Geometry: see drawing. Coordinates: mm, zero at the bounding-box minimum. A direction names the side the tool comes from. Round coordinates to 2 decimals unless told otherwise and drop trailing zeros. Loops run counter-clockwise (first coordinate to the right, second up) from the corner with the lowest first, then second, coordinate; pieces in that order, holes last. Notation, with made-up numbers: (72, 47.5) -> (87, 47.5) arc R8 ccw to (87, 61.5) -> close; hole circle Ø1 at (32.25, 64). An arc over 180 degrees is marked (long way). Answer in a Markdown table with one row per item.
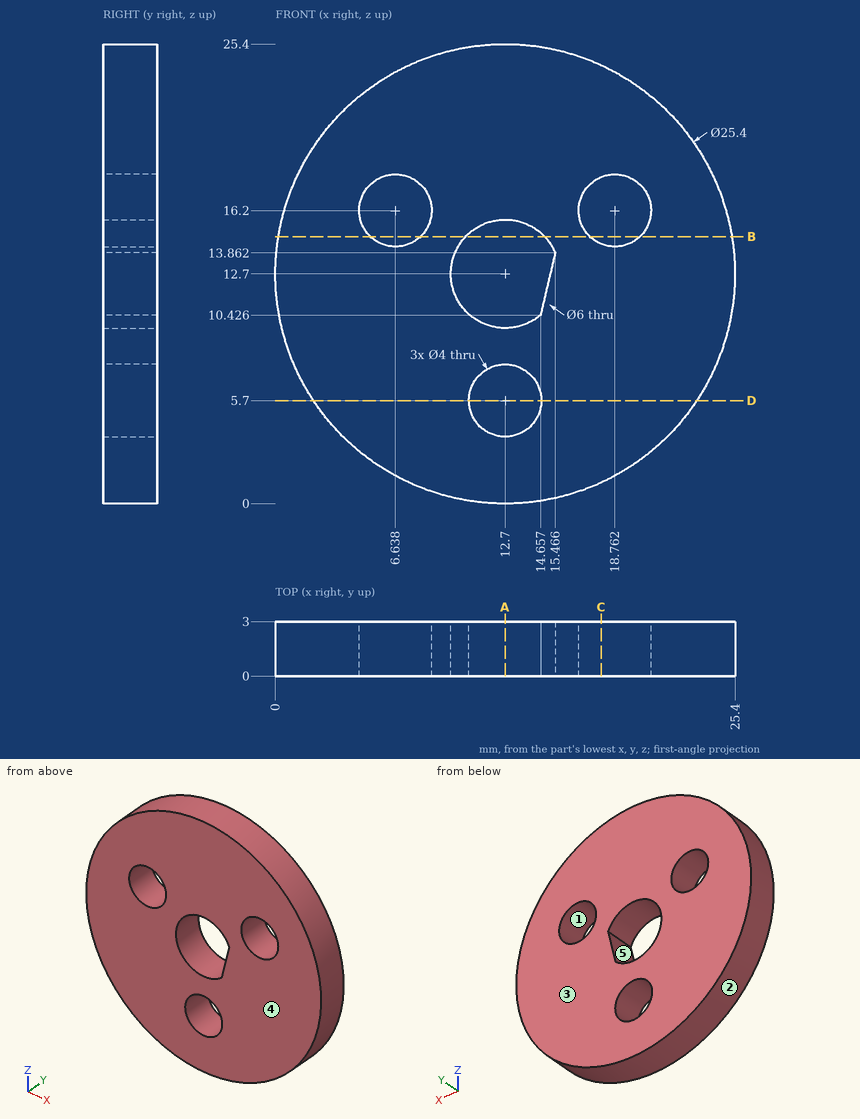
Item 1: Section query C-C, the plane x = 18. Output: boundary loops of the cut face in (y, z).
Ans:
| item | result |
|---|---|
| outline | (0, 1.16) -> (3, 1.16) -> (3, 14.35) -> (0, 14.35) -> close; (0, 18.05) -> (3, 18.05) -> (3, 24.24) -> (0, 24.24) -> close |
Item 2: Section query B-B, the plane z = 14.75. Output: boundary loops of the cut face in (x, y) (1 decimal).
Ans:
| item | result |
|---|---|
| outline | (0.2, 0) -> (5.3, 0) -> (5.3, 3) -> (0.2, 3) -> close; (8, 0) -> (10.5, 0) -> (10.5, 3) -> (8, 3) -> close; (14.9, 0) -> (17.4, 0) -> (17.4, 3) -> (14.9, 3) -> close; (20.1, 0) -> (25.2, 0) -> (25.2, 3) -> (20.1, 3) -> close |
Item 3: Ray query, L1, parallel to X at y = 0.8, z = 16.2; L2, parallel to X at y = 2.3, z = 16 (1 decimal); L3, parallel to X at y = 2.7, z = 15 (1 decimal). Return the intervals inside material, ascending.
Ans:
| item | result |
|---|---|
| L1 | 0.49 to 4.64, 8.64 to 16.76, 20.76 to 24.91 |
| L2 | 0.4 to 4.6, 8.6 to 16.8, 20.8 to 25 |
| L3 | 0.2 to 5, 8.2 to 10.8, 14.6 to 17.2, 20.4 to 25.2 |
Item 4: Set-up query: the marked faces 4 and 5. Return all of +Z, -Z, +X, -X, +Y, -Y with unobstructed straight access to the full face (end or side cutting, diameter ignored); none if empty.
Ans:
| item | result |
|---|---|
| face 4 | +Z, -Z, +X, -X, -Y |
| face 5 | +Y, -Y |
Item 5: Section query D-D, the plane z = 5.7. Output: boundary loops of the cut face in (x, y).
Ans:
| item | result |
|---|---|
| outline | (2.1, 0) -> (10.7, 0) -> (10.7, 3) -> (2.1, 3) -> close; (14.7, 0) -> (23.3, 0) -> (23.3, 3) -> (14.7, 3) -> close |
Item 6: First-contact query: P1, Ø1, axis at y = 0.5, z = 14, coming from the -X side (1 decimal); P2, Ø1, axis at y = 1.5, z = 14.5, coming from the -X side; P3, Ø3, axis at x = 12.7, z = 5.7, coming from the +Y side. Flat tips, straight axial feed; report the tip coordinate or a pass-through.
Ans:
| item | result |
|---|---|
| P1 | x = 0 |
| P2 | x = 0.07 |
| P3 | through |
Item 7: Section query A-A, the plane x = 12.7. Output: boundary loops of the cut face in (y, z), and give its area (3 significant figures).
Ans:
| item | result |
|---|---|
| outline | (0, 0) -> (3, 0) -> (3, 3.7) -> (0, 3.7) -> close; (0, 7.7) -> (3, 7.7) -> (3, 9.7) -> (0, 9.7) -> close; (0, 15.7) -> (3, 15.7) -> (3, 25.4) -> (0, 25.4) -> close |
| area | 46.2 mm2 |
Item 8: Mould query, pull axis X, two halves, no side actions, for the marked faces 1, 2 and 3. Classes: released by +X, released by -X, zero draft, split by the parting line, or undercut.
Ans:
| item | result |
|---|---|
| face 1 | undercut |
| face 2 | split by the parting line |
| face 3 | zero draft |
